Solid Edge part; units mm, degrees
sketch "Sketch1" plane through (0, 0, 0) normal (0, 0, 1) x (1, 0, 0)
  arc A0 (70, 100) -> (80, 90) centre (70, 90) cw
  line L0 (80, 90) -> (80, 10)
  arc A1 (80, 10) -> (70, 0) centre (70, 10) cw
  line L1 (70, 0) -> (0, 0)
  line L2 (0, 0) -> (0, 100)
  line L3 (0, 100) -> (70, 100)
  circle A2 centre (18, 50) radius 16.75
extrude "Protrusion1" add sketch "Sketch1" along normal blind 4
properties material "Acrílico, alto impacto"
Could you check a few things on this model? Use its own coordinates, in mm. Give positions to 0.01 mm unless a question says otherwise; leave off trailing zeros. Order: outer loops, then holes, each group sorted by start corner. A loop starts at its lowest first (then second) coordinate and runs counter-clockwise, first axis right, second up. Notation, with made-up numbers: (56, 21.5) -> (95, 21.5) arc R23 ccw to (95, 41.5) -> close; hole circle Ø6 at (36.5, 77). An arc over 180 degrees is marked (long way). Return JSON: item names as keys, results as strings.
1. Imagine slicing it at A-A on y = 50. List the corners of the cut face in (x, z) for me.
Answer list:
{"outline": "(0, 0) -> (1.25, 0) -> (1.25, 4) -> (0, 4) -> close; (34.75, 0) -> (80, 0) -> (80, 4) -> (34.75, 4) -> close"}
2. Thinking about a two-plate mould opening in X: for faces 1 (the cylindrical face through (33.977, 44.969, 1.972)), 2 (the flat face through (35, 0, 2)), 3 (the flat face through (0, 49, 2)), which applies, pulls with the +X half, pulls with the -X half, needs draft (parallel to the pull), parting line crosses it, or undercut?
Answer list:
{"face 1": "undercut", "face 2": "needs draft", "face 3": "pulls with the -X half"}
3. Imagine slicing it at C-C on z = 1.25. List the corners of the cut face in (x, y) for me.
Answer list:
{"outline": "(0, 0) -> (70, 0) arc R10 ccw to (80, 10) -> (80, 90) arc R10 ccw to (70, 100) -> (0, 100) -> close; hole circle Ø33.5 at (18, 50)"}
4. Imagine slicing it at B-B on x = 18. List the corners of the cut face in (y, z) for me.
Answer list:
{"outline": "(0, 0) -> (33.25, 0) -> (33.25, 4) -> (0, 4) -> close; (66.75, 0) -> (100, 0) -> (100, 4) -> (66.75, 4) -> close"}
5. I need wall thicknesses on line 1 (Y direction, x = 18, z = 3.05); line 2 (Y direction, x = 26.5, z = 2); line 3 (X direction, y = 35, z = 3.7). Which ranges of each line are inside material? Lowest first, please. Write a range as from..to.
Answer list:
{"line 1": "y = 0..33.25, 66.75..100", "line 2": "y = 0..35.57, 64.43..100", "line 3": "x = 0..10.55, 25.45..80"}
